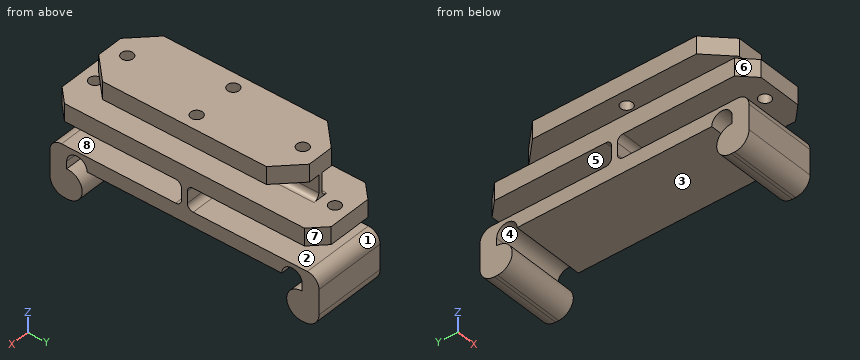
Autodesk Inventor part; units mm, degrees
ref_plane "YZ Plane" through (0, 0, 0) normal (1, 0, 0) x (0, 1, 0)
ref_plane "XZ Plane" through (0, 0, 0) normal (0, 1, 0) x (-1, 0, 0)
ref_plane "XY Plane" through (0, 0, 0) normal (0, 0, 1) x (1, 0, 0)
sketch "Sketch1" plane through (0, 0, 0) normal (1, 0, 0) x (0, 1, 0)
  line L0 (-46, -7.5) -> (-46, 1)
  line L1 (-42, 5) -> (42, 5)
  line L2 (46, 1) -> (46, -7.5)
  line L3 (-41, -12.5) -> (-39.95, -12.5)
  line L4 (-40.25, -2.509) -> (-40.25, 0)
  line L5 (-40.25, 0) -> (40.25, 0)
  line L6 (-1, 5) -> (-1, 13)
  line L7 (-1, 13) -> (1, 13)
  line L8 (1, 13) -> (1, 5)
  line L9 (-46, 19) -> (46, 19)
  line L10 (46, 19) -> (46, 13)
  line L11 (46, 13) -> (-46, 13)
  line L12 (-46, 13) -> (-46, 19)
  arc A0 (46, 1) -> (42, 5) centre (42, 1) ccw
  arc A1 (-42, 5) -> (-46, 1) centre (-42, 1) ccw
  arc A2 (40.25, 0) -> (33.25, 0) centre (36.75, 0) ccw
  arc A3 (-33.25, 0) -> (-40.25, 0) centre (-36.75, 0) ccw
  line L13 (40.25, 0) -> (40.25, -2.509)
  arc A4 (-39.95, -12.5) -> (-40.25, -2.509) centre (-39.95, -7.5) ccw
  arc A5 (-46, -7.5) -> (-41, -12.5) centre (-41, -7.5) ccw
  circle A6 centre (39.95, -7.5) radius 5
  line L14 (41, -12.5) -> (39.95, -12.5)
  arc A7 (41, -12.5) -> (46, -7.5) centre (41, -7.5) ccw
  point P0 (0, 0)
  point P1 (-46, -12.5)
  point P2 (-46, 5)
  point P3 (46, 5)
  point P4 (46, -12.5)
  point P5 (0, 5)
  point P6 (0, 0)
  point P7 (0, 13)
  point P8 (1, 13)
  point P9 (-1, 13)
  point P10 (-40.25, -1.2545)
  point P11 (40.25, -1.2545)
  point P12 (40.25, -2.509)
  dimension "d71" = 10
  dimension "d2" = 80.5
  dimension "d10" = 92
  dimension "d11" = 5
  dimension "d13" = 2
  dimension "d14" = 8
  dimension "d15" = 6
  dimension "d52" = 4
  dimension "d53" = 7
  dimension "d54" = 7
  dimension "d67" = 10
  dimension "d68" = 7.5
  dimension "d69" = 0.3
  dimension "d70" = 5
  dimension "d72" = 0.3
  dimension "d73" = 5
extrude "Extrusion1" add sketch "Sketch1" along normal mid plane 25 contours L0 A1 L1 A0 L2 A7 L14 A6 L13 A2 L5 A3 L4 A4 L3 A5 | L6 L7 L8 L1 | L11 L12 L9 L10 L7 | A6
sketch "Sketch2" plane through (-12.5, -46, 19) normal (0, 0, 1) x (1, 0, 0)
  line L0 (0, 0) -> (25, 0)
  line L1 (25, 92) -> (25, 0)
  line L2 (0, 92) -> (25, 92)
  line L3 (0, 0) -> (0, 92)
  line L4 (13.125, 10) -> (11.875, 10)
  line L5 (11.875, 10) -> (11.875, 82)
  line L6 (11.875, 82) -> (13.125, 82)
  line L7 (13.125, 82) -> (13.125, 10)
  line L8 (13.125, 10) -> (11.875, 82) construction
  line L9 (11.875, 10) -> (13.125, 82) construction
  point P0 (12.5, 46)
  point P1 (20.75, 0)
  point P2 (20.75, 50)
  point P3 (19.25, 50)
  point P4 (19.25, 0)
  point P5 (12.5, 10)
  dimension "d16" = 1.25
  dimension "d19" = 10
extrude "Extrusion2" add sketch "Sketch2" along normal blind 8 contours L4 L5 L6 L7
sketch "Sketch3" plane through (-12.5, -46, 19) normal (0, 0, 1) x (1, 0, 0)
  line L0 (13.125, 82) -> (13.125, 10)
  line L1 (13.125, 10) -> (11.875, 10)
  line L2 (11.875, 10) -> (11.875, 82)
  line L3 (11.875, 82) -> (13.125, 82)
  line L4 (0, 0) -> (25, 0)
  line L5 (25, 92) -> (25, 0)
  line L6 (0, 92) -> (25, 92)
  line L7 (0, 0) -> (0, 92)
  line L8 (13.125, 10) -> (11.875, 10)
  line L9 (12.5, 10) -> (12.5, 0)
  line L10 (11.875, 82) -> (13.125, 82)
  line L11 (12.5, 82) -> (12.5, 92)
  point P0 (12.5, 46)
  point P1 (12.5, 5)
  point P2 (12.5, 87)
hole "Hole1" at (0, -41, 19) at (0, 41, 19) direction (0, 0, -1) diameter 4 depth 8 tip angle 118
sketch "Sketch4" plane through (-12.5, -46, 27) normal (0, 0, 1) x (1, 0, 0)
  line L0 (0, 10) -> (25, 10)
  line L1 (25, 10) -> (25, 82)
  line L2 (25, 82) -> (0, 82)
  line L3 (0, 82) -> (0, 10)
  line L4 (0, 10) -> (25, 82) construction
  line L5 (25, 10) -> (0, 82) construction
  line L6 (13.125, 82) -> (11.875, 82)
  line L7 (0, 0) -> (0, 92)
  point P0 (12.5, 46)
  point P1 (12.5, 82)
  point P2 (0, 46)
extrude "Extrusion3" add sketch "Sketch4" along normal blind 6
sketch "Sketch5" plane through (-12.5, -46, 33) normal (0, 0, 1) x (1, 0, 0)
  line L0 (25, 82) -> (0, 82)
  line L1 (0, 82) -> (0, 10)
  line L2 (0, 10) -> (25, 10)
  line L3 (25, 10) -> (25, 82)
  line L4 (5, 46) -> (20, 46)
  point P0 (12.5, 46)
  point P1 (12.5, 46)
  dimension "d29" = 5
hole "Hole2" at (-7.5, 0, 33) at (7.5, 0, 33) direction (0, 0, -1) diameter 4 depth 8 tip angle 118
sketch "Sketch6" plane through (-12.5, -46, 33) normal (0, 0, 1) x (1, 0, 0)
  circle A0 centre (5, 46) radius 2
  circle A1 centre (20, 46) radius 2
  line L0 (25, 82) -> (0, 82)
  line L1 (0, 82) -> (0, 10)
  line L2 (0, 10) -> (25, 10)
  line L3 (25, 10) -> (25, 82)
  line L4 (12.5, 16) -> (12.5, 76)
  point P0 (12.5, 46)
  point P1 (12.5, 46)
  point P2 (12.5, 46)
  dimension "d38" = 60
hole "Hole3" at (0, -30, 33) at (0, 30, 33) direction (0, 0, -1) diameter 4 depth 5
chamfer "Chamfer1" distance 5 angle 45 4 edges at (-12.5, -46, 16) (-12.5, 46, 16) (12.5, -46, 16) (12.5, 46, 16)
chamfer "Chamfer2" distance 8 angle 45 4 edges at (12.5, 36, 30) (12.5, -36, 30) (-12.5, -36, 30) (-12.5, 36, 30)
fillet "Fillet1" radius 2 6 edges at (0.625, 0, 19) (-0.625, 0, 19) (0, -1, 5) (0, 1, 5) (0, -1, 13) (0, 1, 13)
properties part number "Rail-FlextureBase" material "ABS Plastic"
Model file for the job. Use its own axes, mm. Face numbers are marked on the shaded views. A direction names the side the tool comes from. Give positions to 0.01 mm unless a question says otherwise; leave off trailing zeros. Order: outer loops, then holes, each group sorted by start corner. A loop starts at its lowest first (then second) coordinate and runs counter-clockwise, first axis right, second up. Notation, with made-up numbers: M 20,33 L 68,33 A22 ccw 68,67 Z; hole C 74.25,79.25 d1. An arc over 180 degrees is marked long. Put each result on its own line as item: value. Start each with the question number.
(1) Band-saw the part on B-B on z = 29. Give the cut face in (x, y).
(2) Pull direction Y, two halves, no side cores. Call the marked faces 1, 2, 3 and 4: released by +Y, released by -Y, zero draft, split by the parting line, or undercut.
(3) Band-saw the part on D-D on y = 18.5. Give the cut face in (x, z) (3 decimals), then the cut area to 3 significant figures.
(4) Pin check, flat tips, straight feed: pin 1 Ø10 at (y, z) = (17.5, -6.5) entering from +X; pin 2 Ø10 at (x, z) = (-1.5, 28) entering from -Y; pin 3 Ø12 at (x, y) = (5, -19.5) entering from -Z; pin 4 Ø1 at (x, z) = (-1, 11) entering from +Y. Stop position of each tip, or through.
(5) Band-saw the part on C-C on z = 2. Give the cut face in (x, y), then the cut area to 3 significant figures.
(6) Drill centre lines: L1, parallel to X at y = 0, z = 29; L2, parallel to Z at x = -10.5, y = 15; L3, parallel to Y at x = 0, z = 16.3. Where is each one in solid material? Low to high. Write a range as [from, to].
(7) Band-saw the part on A-A on y = -30. Give the cut face in (x, z) (3 decimals), then the cut area to 3 significant figures.
(8) Tool access for the marked faces 5, 6, 7 and 8: list every direction of +Z, -Z, +X, -X, +Y, -Y with a clear straight run to the whole face (end or side of a thin tool).
Results below:
1. outline: M -12.5,-28 L -4.5,-36 L 4.5,-36 L 12.5,-28 L 12.5,28 L 4.5,36 L -4.5,36 L -12.5,28 Z; hole C -7.5,0 d4; hole C 0,-30 d4; hole C 0,30 d4; hole C 7.5,0 d4
2. face 1: released by +Y
2. face 2: zero draft
2. face 3: undercut
2. face 4: undercut
3. outline: M -12.5,0 L 12.5,0 L 12.5,5 L -12.5,5 Z; M -12.5,13 L 12.5,13 L 12.5,19 L 2.625,19 A2 cw 0.625,21 L 0.625,27 L 12.5,27 L 12.5,33 L -12.5,33 L -12.5,27 L -0.625,27 L -0.625,21 A2 cw -2.625,19 L -12.5,19 Z
3. area: 437 mm2
4. pin 1: passes through
4. pin 2: stops at y = -36
4. pin 3: stops at z = 0
4. pin 4: stops at y = 1.06
5. outline: M -12.5,-45.87 L 12.5,-45.87 L 12.5,-39.62 L -12.5,-39.62 Z; M -12.5,-33.88 L 12.5,-33.88 L 12.5,33.88 L -12.5,33.88 Z; M -12.5,39.62 L 12.5,39.62 L 12.5,45.87 L -12.5,45.87 Z
5. area: 2,010 mm2
6. L1: x = [-12.5, -9.5], [-5.5, 5.5], [9.5, 12.5]
6. L2: z = [0, 5], [13, 19], [27, 33]
6. L3: y = [-46, -43], [-39, 39], [43, 46]
7. outline: M -12.5,0 L 12.5,0 L 12.5,5 L -12.5,5 Z; M -12.5,13 L 12.5,13 L 12.5,19 L 2.625,19 A2 cw 0.625,21 L 0.625,27 L 10.5,27 L 10.5,33 L 2,33 L 2,28 L -2,28 L -2,33 L -10.5,33 L -10.5,27 L -0.625,27 L -0.625,21 A2 cw -2.625,19 L -12.5,19 Z
7. area: 393 mm2
8. face 5: +X, -X, +Y
8. face 6: +Z, -X, -Y
8. face 7: +Z, +X, +Y
8. face 8: +X, -X, -Y
